Input: part model. Units: mm. Frame: model coordinates. A direction names the side the tool comes from. Round coordinates to 2 decimals unless told otherwise and drop trailing zeros. Loops run counter-clockwise (first coordinate to the right, second up) from the corner with the lowest first, then second, coordinate; pieces in that order, holes last. Notation, with made-up numbers: (46, 23) -> (76, 23) arc R25 cw to (76, 60) -> close; hole circle Ø10 at (-17, 19.25). An arc over 180 degrees is marked (long way). Answer in a Markdown table with one row per item. Add a question column.
Q1. Reachability of faces 1 (the face through (31.734, 28.776, -25.143)), 2 (the face through (-34, 19, -25)), 3 (the face through (31, 12, 0)), 4 (the face through (31, 17, -64)), 5 (the face through (64, 32, -32)) from +Z, -Z, +X, -X, +Y, -Y: full face, straight path, thin tool, end or side. Return the list, or none.
Q2. Section A-A, the plane z = -32. Output: boundary loops of the cut face in (x, y).
Q3. Ray query, L1, parallel to X at y = 10, z = -32; L2, parallel to X at y = 40.5, z = -24.5; L3, parallel to X at y = 12, z = -41.5. Return the intervals inside material, ascending. Write a range as from..to.
Q4. Pin query (flat end, axial travel): pin 1 (5 mm diameter, centred on y = 20.5, z = -52, fed in from -X); pin 2 (4 mm diameter, centred on y = 30.5, z = -26, fed in from -X); pin 3 (17 mm diameter, centred on x = 90.5, z = -26, fed in from +Y). Return the tip coordinate at first contact, or that it passes through.
Q5. Section C-C, the plane y = 6. Output: boundary loops of the cut face in (x, z).
Q6. Mould query, pull axis Z, two halves, no side actions, for faces 6 (the face through (120.992, 9.367, -32.704)), 7 (the face through (-29.213, 9.367, -21.839)), 8 (the face through (31, 0, -32)). Classes: pulls with the +Z half, pulls with the -Z half, needs draft (parallel to the pull), parting line crosses it, or undercut.
Q7. Section B-B, the plane x = 19. Output: boundary loops of the cut face in (y, z), and give its area (3 significant figures).
Q8. Section D-D, the plane x = 96.5. Output: boundary loops of the cut face in (y, z), and give its area (3 significant figures).
```python
from build123d import *

# Parameters (mm, degrees)
SKETCH1_W           = 64
SKETCH1_H           = 64
BOSS_EXTRUDE1_DEPTH = 45
SKETCH2_R           = 11
BOSS_EXTRUDE4_DEPTH = 19
SKETCH10_W          = 38
SKETCH10_H          = 51
CUT_EXTRUDE5_DEPTH  = 63
SKETCH12_W          = 38
SKETCH12_H          = 51
BOSS_EXTRUDE5_DEPTH = 13
BOSS_EXTRUDE6_DEPTH = 47


with BuildPart() as part:
    # Sketch1 → Boss-Extrude1 (new body)
    with BuildSketch(Plane(origin=(0, 0, 0), x_dir=(1, 0, 0), z_dir=(0, 1, 0))):
        with Locations((32, 32)):
            Rectangle(SKETCH1_W, SKETCH1_H)
    extrude(amount=BOSS_EXTRUDE1_DEPTH)

    # Sketch2 → Boss-Extrude4 (add)
    # profile 1 of 2: a face of its own
    with BuildSketch(Plane(origin=(0, 0, 0), x_dir=(1, 0, 0), z_dir=(0, 1, 0))):
        with BuildLine():
            Line((0, 64), (0, 0))
            Line((0, 0), (-25, 0))
            ThreePointArc((-25, 0), (-57, 32), (-25, 64))
            Line((-25, 64), (0, 64))
        make_face()
        with Locations(Location((-25, 32, 0), (0, 0, 270))):
            Circle(SKETCH2_R, mode=Mode.SUBTRACT)
    # profile 2 of 2: a face of its own
    with BuildSketch(Plane(origin=(0, 0, 0), x_dir=(1, 0, 0), z_dir=(0, 1, 0))):
        with BuildLine():
            Line((89, 0), (64, 0))
            Line((64, 0), (64, 64))
            Line((64, 64), (89, 64))
            ThreePointArc((89, 64), (121, 32), (89, 0))
        make_face()
        with Locations(Location((89, 32, 0), (0, 0, 270))):
            Circle(SKETCH2_R, mode=Mode.SUBTRACT)
    extrude(amount=BOSS_EXTRUDE4_DEPTH)

    # Sketch10 → Cut-Extrude5 (cut)
    with BuildSketch(Plane(origin=(0, 0, 0), x_dir=(1, 0, 0), z_dir=(0, 1, 0))):
        with Locations((32, 25.5)):
            Rectangle(SKETCH10_W, SKETCH10_H)
    extrude(amount=CUT_EXTRUDE5_DEPTH, mode=Mode.SUBTRACT)

    # Sketch12 → Boss-Extrude5 (add)
    with BuildSketch(Plane(origin=(0, 0, 0), x_dir=(1, 0, 0), z_dir=(0, 1, 0))):
        with Locations((32, 25.5)):
            Rectangle(SKETCH12_W, SKETCH12_H)
    extrude(amount=BOSS_EXTRUDE5_DEPTH)

    # Sketch13 → Boss-Extrude6 (add)
    with BuildSketch(Plane(origin=(13, 0, 0), x_dir=(0, 0, -1), z_dir=(1, 0, 0))):
        Polygon((0, 13), (51, 45), (51, 13), align=None)
    extrude(amount=BOSS_EXTRUDE6_DEPTH)


solid = part.part
```
Answer block:
| question | item | result |
|---|---|---|
| 1 | face 1 | +Z, +Y |
| 1 | face 2 | +Z, -Z, -X, +Y |
| 1 | face 3 | +Z, +X, -X, +Y, -Y |
| 1 | face 4 | -Z, +X, -X, +Y, -Y |
| 1 | face 5 | +Z, -Z, +X, +Y |
| 2 | outline | (-57, 0) -> (-36, 0) -> (-36, 19) -> (-57, 19) -> close; (-14, 0) -> (78, 0) -> (78, 19) -> (64, 19) -> (64, 45) -> (51, 45) -> (51, 33.08) -> (13, 33.08) -> (13, 45) -> (0, 45) -> (0, 19) -> (-14, 19) -> close; (100, 0) -> (121, 0) -> (121, 19) -> (100, 19) -> close |
| 3 | L1 | -57..-36, -14..78, 100..121 |
| 3 | L2 | 0..13, 51..64 |
| 3 | L3 | -55.56..-30.55, -19.45..83.45, 94.55..119.56 |
| 4 | pin 1 | x = -51.46 |
| 4 | pin 2 | x = 0 |
| 4 | pin 3 | y = 19 |
| 5 | outline | (-25, -64) -> (89, -64) arc R32 ccw to (89, 0) -> (-25, 0) arc R32 ccw to start; hole circle Ø22 at (-25, -32); hole circle Ø22 at (89, -32) |
| 6 | face 6 | parting line crosses it |
| 6 | face 7 | undercut |
| 6 | face 8 | needs draft |
| 7 | outline | (0, -64) -> (45, -64) -> (45, -51) -> (13, 0) -> (0, 0) -> close |
| 7 | area | 2,060 mm^2 |
| 8 | outline | (0, -63.11) -> (19, -63.11) -> (19, -40.05) -> (0, -40.05) -> close; (0, -23.95) -> (19, -23.95) -> (19, -0.89) -> (0, -0.89) -> close |
| 8 | area | 876 mm^2 |
